Geometry check sheet. Reference: the model listing, model coordinates, mm. Face numbers are marked on the shaded views. A direction names the side the tool comes from. Round coordinates to 2 decimals unless told otherwise and drop trailing zeros. Write each loop counter-clockwise with the first axis right and the second up, starting at its lowest first coordinate (ties: lowest second). Pieces come first, ordered by that corner, then holes.
from build123d import *

# Parameters (mm, degrees)
SKETCH1_R           = 14
BOSS_EXTRUDE2_DEPTH = 19
BOSS_EXTRUDE4_START = -0.7
SKETCH2_R           = 2.1
BOSS_EXTRUDE4_DEPTH = 0.7
BOSS_EXTRUDE5_START = -16
BOSS_EXTRUDE5_DEPTH = 16
SKETCH4_R           = 4.5
BOSS_EXTRUDE6_DEPTH = 1.5
SKETCH5_R           = 2.5
BOSS_EXTRUDE7_DEPTH = 8.5
CUT_EXTRUDE1_START  = -6
CUT_EXTRUDE1_DEPTH  = 6


with BuildPart() as part:
    # Sketch1 → Boss-Extrude2 (new body)
    with BuildSketch(Plane(origin=(0, 0, 0), x_dir=(1, 0, 0), z_dir=(0, 1, 0))):
        with Locations(Location((0, 0, 0), (0, 0, 270))):
            Circle(SKETCH1_R)
    extrude(amount=BOSS_EXTRUDE2_DEPTH)

    # Sketch2 → Boss-Extrude4 (add)
    # profile 1 of 2: a face of its own
    with BuildSketch(Plane(origin=(0, 19, 0), x_dir=(1, 0, 0), z_dir=(0, 1, 0)).offset(BOSS_EXTRUDE4_START)):
        with BuildLine():
            Line((17.5, 3.5), (13.555441712, 3.5))
            ThreePointArc((13.555441712, 3.5), (13.888415748, 1.764060095), (14, 0))
            ThreePointArc((14, 0), (13.888415748, -1.764060095), (13.555441712, -3.5))
            Line((13.555441712, -3.5), (17.5, -3.5))
            ThreePointArc((17.5, -3.5), (21, 0), (17.5, 3.5))
        make_face()
        with Locations(Location((17.5, 0, 0), (0, 0, 270))):
            Circle(SKETCH2_R, mode=Mode.SUBTRACT)
    # profile 2 of 2: a face of its own
    with BuildSketch(Plane(origin=(0, 19, 0), x_dir=(1, 0, 0), z_dir=(0, 1, 0)).offset(BOSS_EXTRUDE4_START)):
        with BuildLine():
            Line((-13.555441712, 3.5), (-17.5, 3.5))
            ThreePointArc((-17.5, 3.5), (-21, 0), (-17.5, -3.5))
            Line((-17.5, -3.5), (-13.555441712, -3.5))
            ThreePointArc((-13.555441712, -3.5), (-14, 0), (-13.555441712, 3.5))
        make_face()
        with Locations(Location((-17.5, 0, 0), (0, 0, 270))):
            Circle(SKETCH2_R, mode=Mode.SUBTRACT)
    extrude(amount=BOSS_EXTRUDE4_DEPTH)

    # Sketch3 → Boss-Extrude5 (add)
    with BuildSketch(Plane(origin=(0, 19, 0), x_dir=(1, 0, 0), z_dir=(0, 1, 0)).offset(BOSS_EXTRUDE5_START)):
        with BuildLine():
            Line((-7.3, -11.94612908), (-7.3, -17))
            Line((-7.3, -17), (7.3, -17))
            Line((7.3, -17), (7.3, -11.94612908))
            ThreePointArc((7.3, -11.94612908), (0, -14), (-7.3, -11.94612908))
        make_face()
    extrude(amount=BOSS_EXTRUDE5_DEPTH)

    # Sketch4 → Boss-Extrude6 (add)
    with BuildSketch(Plane(origin=(0, 19, 0), x_dir=(1, 0, 0), z_dir=(0, 1, 0))):
        with Locations(Location((0, 8, 0), (0, 0, 270))):
            Circle(SKETCH4_R)
    extrude(amount=BOSS_EXTRUDE6_DEPTH)

    # Sketch5 → Boss-Extrude7 (add)
    with BuildSketch(Plane(origin=(0, 20.5, 0), x_dir=(1, 0, 0), z_dir=(0, 1, 0))):
        with Locations(Location((0, 8, 0), (0, 0, 270))):
            Circle(SKETCH5_R)
    extrude(amount=BOSS_EXTRUDE7_DEPTH)

    # Sketch7 → Cut-Extrude1 (cut)
    with BuildSketch(Plane(origin=(0, 29, 0), x_dir=(1, 0, 0), z_dir=(0, 1, 0)).offset(CUT_EXTRUDE1_START)):
        with BuildLine():
            Line((-2, 9.5), (2, 9.5))
            ThreePointArc((2, 9.5), (0, 10.5), (-2, 9.5))
        make_face()
        with BuildLine():
            Line((-2, 6.5), (2, 6.5))
            ThreePointArc((2, 6.5), (0, 5.5), (-2, 6.5))
        make_face()
    extrude(amount=CUT_EXTRUDE1_DEPTH, mode=Mode.SUBTRACT)


solid = part.part
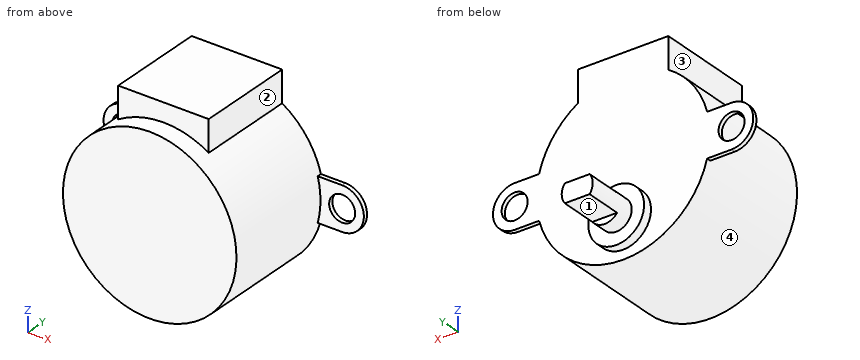
1. Access from +Z, -Z, +X, -X, +Y, -Y to the whole of each face (thin tool, end or side, straight path). Record for the marked faces 1, 2, 3 and 4.
2. Section check A-A (z = 0). Record the cut outline in (x, y).
3. Section check B-B (x = -18). Record the cut outline in (y, z), plus the area to 3 significant figures.
4. Scan lines: line 1 along X through (y, z) = (18.5, 0); line 2 along Y through (x, z) = (10.5, 6); line 3 along Y through (x, z) = (-1, -4). Record each from-to range of solid material in increasing order.
5. Depth check by flat-ended pin: pin 1 Ø3 at (x, y) = (0, 27) entering from +Z; pin 2 Ø1.5 at (y, z) = (13.5, 15) entering from -X; pin 3 Ø2.5 at (y, z) = (11.5, 14.5) entering from +X; pin 4 Ø2 at (x, z) = (-17.5, -1) entering from -Y. Enter the tip coordinate at first touch or a pass-through.
6. Section check D-D (z = -8). Record the cut outline in (x, y), plus the area to 3 significant figures.
7. Section check C-C (x = 0). Record the cut outline in (y, z).
Results below:
1. face 1: -Z, +X, -X, +Y
1. face 2: +Z, +X, +Y, -Y
1. face 3: +Z, -X, +Y, -Y
1. face 4: -Y
2. outline: (-21, 18.3) - (-19.6, 18.3) - (-19.6, 19) - (-21, 19) - close; (-15.4, 18.3) - (-14, 18.3) - (-14, 0) - (14, 0) - (14, 18.3) - (15.4, 18.3) - (15.4, 19) - (-15.4, 19) - close; (19.6, 18.3) - (21, 18.3) - (21, 19) - (19.6, 19) - close
3. outline: (18.3, -3.46) - (19, -3.46) - (19, -2.04) - (18.3, -2.04) - close; (18.3, 2.04) - (19, 2.04) - (19, 3.46) - (18.3, 3.46) - close
3. area: 1.99 mm2
4. line 1: x = -21 to -19.6, -15.4 to 15.4, 19.6 to 21
4. line 2: y = 0 to 19
4. line 3: y = 0 to 20.5
5. pin 1: stops at z = -6.5
5. pin 2: stops at x = -7.3
5. pin 3: stops at x = 7.3
5. pin 4: passes through
6. outline: (-11.49, 0) - (11.49, 0) - (11.49, 19) - (4.5, 19) - (4.5, 20.5) - (2.5, 20.5) - (2.5, 29) - (-2.5, 29) - (-2.5, 20.5) - (-4.5, 20.5) - (-4.5, 19) - (-11.49, 19) - close
6. area: 493 mm2
7. outline: (0, -14) - (19, -14) - (19, -12.5) - (20.5, -12.5) - (20.5, -10.5) - (23, -10.5) - (23, -9.5) - (29, -9.5) - (29, -6.5) - (23, -6.5) - (23, -5.5) - (20.5, -5.5) - (20.5, -3.5) - (19, -3.5) - (19, 17) - (3, 17) - (3, 14) - (0, 14) - close
